Can you work these out from the model? Positions are in its coordinate system, mm. A direction names the side the tool comes from. Give positions to 0.01 mm unless a question says otherwise; leave off trailing zeros. Order: outer loops, then holes, each group sorted by start corner. A loop starts at its lowest first (then second) coordinate and runs counter-clockwise, first axis right, second up. Notation, with made-up numbers: (24.5, 33) -> (38.5, 33) arc R23 ccw to (38.5, 61) -> close; hole circle Ø10 at (61.5, 41.5). An arc over 180 degrees is marked (long way). Answer as CSV lines item,"result".
```python
from build123d import *

# Parameters (mm, degrees)
SKETCH1_W           = 12.7
SKETCH1_H           = 10.16
SKETCH3_W           = 25.4
SKETCH3_H           = 25.4
BOSS_EXTRUDE2_DEPTH = 12.7


with BuildPart() as part:
    # Sketch1 → Revolve3 (revolve)
    with BuildSketch(Plane.XY, mode=Mode.PRIVATE) as revolve3_sk:
        Polygon((101.6, 19.05), (0, 19.05), (0, 0), (152.4, 0), (152.4, 10.16), align=None)
        with Locations((158.75, 5.08)):
            Rectangle(SKETCH1_W, SKETCH1_H)
    revolve(revolve3_sk.sketch.rotate(Axis((0, 0, 0), (1, 0, 0)), 180), axis=Axis((0, 0, 0), (1, 0, 0)))

    # Sketch3 → Boss-Extrude2 (add)
    with BuildSketch(Plane(origin=(165.1, 0, 0), x_dir=(0, 0, -1), z_dir=(1, 0, 0))):
        Rectangle(SKETCH3_W, SKETCH3_H)
    extrude(amount=BOSS_EXTRUDE2_DEPTH)

    # Mirror1: part across plane


with BuildPart() as part_1:
    add(part.part)
    add(part.part.mirror(Plane(origin=(0, 0, 0), x_dir=(0, 0, 1), z_dir=(1, 0, 0))))


solid = part_1.part
```
Item 1: For pin 1 (10 mm diameter, centred on x = 63.5, z = -12.5, fed in from -Y); pin 2 (10 mm diameter, centred on x = 169, y = -2, fed in from -Z); pin 3 (10 mm diameter, centred on x = -172.5, z = -2, fed in from -Y), each with a flat end and sliding along its axis, tell me the tip position at first contact or that it passes through.
Numbers:
pin 1,"stops at y = -17.51"
pin 2,"stops at z = -12.7"
pin 3,"stops at y = -12.7"
Item 2: Imagine slicing it at C-C, the plane x = 58. Please give me the cut outline in (y, z), then the cut area to 3 significant figures.
Numbers:
outline,"circle Ø38.1 at (0, 0)"
area,"1,140 mm²"
Item 3: We'd pull the mould along X, two halves only. Please class faces 5 (the cylindrical face through (-158.839, 1.323, -10.074)), 6 (the flat face through (171, 0, -12.7)), 7 (the flat face through (-165.1, 9, 6)), 8 (the flat face through (177.8, 0, 0)): released by +X, released by -X, zero draft, split by the parting line, or undercut.
Numbers:
face 5,"undercut"
face 6,"zero draft"
face 7,"undercut"
face 8,"released by +X"
Item 4: For faces 1 (the flat face through (-171, -12.7, 0)), 2 (the conical face through (126.644, 11.639, 8.925)), 3 (the flat face through (-171, 0, 12.7)), 4 (the flat face through (171, -12.7, 0)), which set-ups out of +Z, -Z, +X, -X, +Y, -Y let a thin tool reach every point of the face, with its end or its side?
Numbers:
face 1,"+Z, -Z, -X, -Y"
face 2,"none"
face 3,"+Z, -X, +Y, -Y"
face 4,"+Z, -Z, +X, -Y"
Item 5: Please list where these lines run through material, in increasing order: line 1 along Y through (x, z) = (57.5, 12.5); line 2 along Y through (x, z) = (-35.5, 17.5); line 3 along Z through (x, y) = (96, -6).
Numbers:
line 1,"y = -14.38 to 14.38"
line 2,"y = -7.53 to 7.53"
line 3,"z = -18.08 to 18.08"
